```python
from build123d import *

# Parameters (mm, degrees)
SKETCH_W              = 115
SKETCH_H              = 25
PAD_DEPTH             = 3
PAD001_DEPTH          = 3
SKETCH002_W           = 115
SKETCH002_H           = 25
SKETCH002_W_2         = 96
SKETCH002_H_2         = 3
PAD002_DEPTH          = 3
SKETCH003_R           = 0.825
POCKET_DEPTH          = 245.060315
POLARPATTERN_COUNT    = 2
POLARPATTERN001_COUNT = 2
POLARPATTERN002_COUNT = 2
FILLET_R              = 2
SKETCH004_R           = 12.75
POCKET001_DEPTH       = 3
POCKET002_DEPTH       = 3
FILLET001_R           = 0.4
FILLET002_R           = 2


with BuildPart() as part:
    # Sketch → Pad (new body)
    with BuildSketch(Plane.XY):
        Rectangle(SKETCH_W, SKETCH_H)
    extrude(amount=PAD_DEPTH)

    # Sketch001 (on Face6 of Pad) → Pad001 (join)
    with BuildSketch(Plane.XY.offset(3)):
        Polygon((-57.5, 12.5), (57.5, 12.5), (57.5, 4), (50, 4), (50, 5), (-50, 5), (-50, 4), (-57.5, 4), align=None)
        Polygon((-57.5, -12.5), (57.5, -12.5), (57.5, -4), (50, -4), (50, -5), (-50, -5), (-50, -4), (-57.5, -4), align=None)
    extrude(amount=PAD001_DEPTH)

    # Sketch002 (on Face12 of Pad001) → Pad002 (join)
    with BuildSketch(Plane.XY.offset(6)):
        Rectangle(SKETCH002_W, SKETCH002_H)
        Rectangle(SKETCH002_W_2, SKETCH002_H_2, mode=Mode.SUBTRACT)
    extrude(amount=PAD002_DEPTH)

    # Sketch003 (on Face26 of Pad002) → Pocket (cut, through all)
    with BuildSketch(Plane.XY.offset(9)):
        with Locations((-52.5, 7.5)):
            Circle(SKETCH003_R)
    pocket = extrude(amount=-POCKET_DEPTH, mode=Mode.SUBTRACT)

    # PolarPattern: Pocket ×2 about axis
    polarpattern_axis = Axis((0, 0, 0), (0, 1, 0))
    for i in range(1, POLARPATTERN_COUNT):
        add(pocket.rotate(polarpattern_axis, i * 360 / POLARPATTERN_COUNT), mode=Mode.SUBTRACT)

    # PolarPattern001: Pocket ×2 about axis
    polarpattern001_axis = Axis((0, 0, 0), (1, 0, 0))
    for i in range(1, POLARPATTERN001_COUNT):
        add(pocket.rotate(polarpattern001_axis, i * 360 / POLARPATTERN001_COUNT), mode=Mode.SUBTRACT)

    # PolarPattern002: Pocket ×2 about axis
    polarpattern002_axis = Axis((0, 0, 9), (0, 0, 1))
    for i in range(1, POLARPATTERN002_COUNT):
        add(pocket.rotate(polarpattern002_axis, i * 360 / POLARPATTERN002_COUNT), mode=Mode.SUBTRACT)

    # Fillet
    fillet_edges = [part.edges().sort_by_distance(p)[0] for p in [
        (57.5, 12.5, 7.5),
        (57.5, 12.5, 4.5),
        (57.5, 12.5, 1.5),
        (57.5, -12.5, 7.5),
        (-57.5, 12.5, 7.5),
        (-57.5, -12.5, 7.5),
    ]]
    fillet(fillet_edges, radius=FILLET_R)

    # Sketch004 (on Face2 of Fillet) → Pocket001 (cut)
    with BuildSketch(Plane(origin=(0, 0, 0), x_dir=(1, 0, 0), z_dir=(0, 0, -1))):
        with Locations((0, -4.31247)):
            Circle(SKETCH004_R)
    extrude(amount=-POCKET001_DEPTH, mode=Mode.SUBTRACT)

    # Sketch005 (on Face2 of Pocket001) → Pocket002 (cut)
    with BuildSketch(Plane(origin=(0, 0, 0), x_dir=(1, 0, 0), z_dir=(0, 0, -1))):
        Polygon((0.086598, 10.584693), (-50.025204, 10.584693), (-50.025204, 6.371434), (-55.624748, 3.161258), (-55.624748, -3.408425), (-50.493088, -3.376352), (-45.134857, 4.115264), (-43.691578, 5.783052), (0.086598, 5.783052), align=None)
    extrude(amount=-POCKET002_DEPTH, mode=Mode.SUBTRACT)

    # Fillet001
    fillet001_edges = [part.edges().sort_by_distance(p)[0] for p in [
        (-7.787357, -5.783052, 1.5),
    ]]
    fillet(fillet001_edges, radius=FILLET001_R)

    # Fillet002
    fillet002_edges = [part.edges().sort_by_distance(p)[0] for p in [
        (0.086598, -8.437236, 1.5),
    ]]
    fillet(fillet002_edges, radius=FILLET002_R)


solid = part.part
```
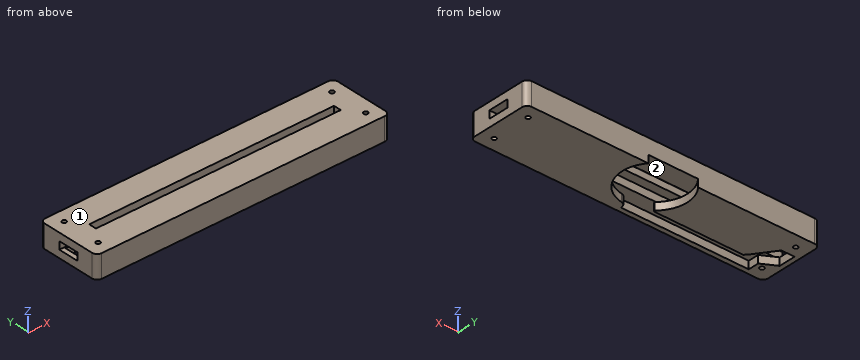
Design review of the part built by this model. Coordinates are the model's own, in mm. Face numbers are marked on the shaded views. Round coordinates to 2 decimals unless told otherwise and drop trailing zeros. Order: outer loops, then holes, each group sorted by start corner. A loop starts at its lowest first (then second) coordinate and runs counter-clockwise, first axis right, second up. Notation, with made-up numbers: (57, 80.5) - (65, 80.5) arc R15 cw to (65, 90.5) - close; hole circle Ø3 at (-19, -8.5). An arc over 180 degrees is marked (long way). One line per question, with ' | ' between items.
Item 1: Draft analysis for pull direction X (two halves, no side actions). For the marked faces 1 and 2, state which applies: +X half, -X half, draft (parallel to the pull), parting line (faces both ways), or undercut.
Checks:
face 1: draft | face 2: undercut
Item 2: Take a section at B-B, the plane x = 40. Write out the cut boundary in (y, z), then the cut area to 3 significant figures.
Checks:
outline: (-12.5, 0) - (12.5, 0) - (12.5, 9) - (1.5, 9) - (1.5, 6) - (5, 6) - (5, 3) - (-5, 3) - (-5, 6) - (-1.5, 6) - (-1.5, 9) - (-12.5, 9) - close | area: 186 mm²
Item 3: Wall thickness on line 1 (Y direction, x = -52.5, z = 7.25) (3 decimals); line 2 (Y direction, x = -52.5, z = 4.5) (3 decimals); line 3 (X direction, y = -7.5, z = 3.5) (3 decimals): over which ranges is each line inside the solid? List them lowest first. Write a range as [from, to].
Checks:
line 1: [-12.5, -8.325], [-6.675, 6.675], [8.325, 12.5] | line 2: [-12.5, -8.325], [-6.675, -4], [4, 6.675], [8.325, 12.5] | line 3: [-57.5, -53.325], [-51.675, 51.675], [53.325, 57.5]
Item 4: For P1, Ø5, axis at x = -23, y = 0.5, coming from the +Z side; P2, Ø1.5, axis at x = 52.5, y = 7.5, coming from the +Z side; P3, Ø5, axis at x = -4.5, y = 0.5, coming from the -Z side; P4, Ø2.5, axis at x = 5, y = 7.5, coming from the -Z side, all flat-tipped, find the tip position at first contact; note any pin that passes through.
Checks:
P1: z = 9 | P2: through | P3: z = 6 | P4: z = 3
Item 5: Take a section at A-A, the plane z = 4.5. Write out the cut boundary in (x, y) (3 decimals).
Checks:
outline: (-57.5, -10.5) arc R2 ccw to (-55.5, -12.5) - (55.5, -12.5) arc R2 ccw to (57.5, -10.5) - (57.5, -4) - (50, -4) - (50, -5) - (-50, -5) - (-50, -4) - (-57.5, -4) - close; (-57.5, 4) - (-50, 4) - (-50, 5) - (50, 5) - (50, 4) - (57.5, 4) - (57.5, 10.5) arc R2 ccw to (55.5, 12.5) - (-55.5, 12.5) arc R2 ccw to (-57.5, 10.5) - close; hole circle Ø1.65 at (-52.5, -7.5); hole circle Ø1.65 at (-52.5, 7.5); hole circle Ø1.65 at (52.5, -7.5); hole circle Ø1.65 at (52.5, 7.5)
